```python
from build123d import *

# Parameters (mm, degrees)
SKETCH_2_W          = 308
SKETCH_2_H          = 840
EXTRUDE_1_DEPTH     = 1
SKETCH_2_3_W        = 22
SKETCH_2_3_H        = 840
EXTRUDE_2_DEPTH     = 22
SKETCH_4_W          = 20
SKETCH_4_H          = 20
CUT_EXTRUDE_1_DEPTH = 840
SKETCH_4_3_W        = 20
SKETCH_4_3_H        = 20
CUT_EXTRUDE_2_DEPTH = 840


with BuildPart() as part:
    # 스케치2 → 보스-돌출1 (new body)
    with BuildSketch(Plane.XY):
        with Locations((-176, 420)):
            Rectangle(SKETCH_2_W, SKETCH_2_H)
    extrude(amount=EXTRUDE_1_DEPTH)

    # 스케치2<3> → 보스-돌출2 (add)
    with BuildSketch(Plane.XY):
        with Locations((-11, 420)):
            Rectangle(SKETCH_2_3_W, SKETCH_2_3_H)
        with Locations((-341, 420)):
            Rectangle(SKETCH_2_3_W, SKETCH_2_3_H)
    extrude(amount=EXTRUDE_2_DEPTH)

    # 스케치4 → 컷-돌출1 (cut)
    with BuildSketch(Plane(origin=(0, 840, 0), x_dir=(1, 0, 0), z_dir=(0, 1, 0))):
        with Locations((-11, -11)):
            Rectangle(SKETCH_4_W, SKETCH_4_H)
    extrude(amount=-CUT_EXTRUDE_1_DEPTH, mode=Mode.SUBTRACT)

    # 스케치4<3> → 컷-돌출2 (cut)
    with BuildSketch(Plane(origin=(0, 840, 0), x_dir=(1, 0, 0), z_dir=(0, 1, 0))):
        with Locations((-341, -11)):
            Rectangle(SKETCH_4_3_W, SKETCH_4_3_H)
    extrude(amount=-CUT_EXTRUDE_2_DEPTH, mode=Mode.SUBTRACT)


solid = part.part
```
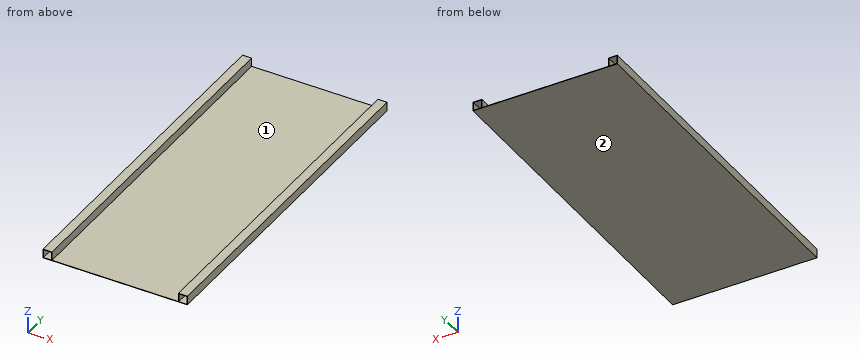
Check sheet for the modelled part. Datum: model origin and axes. Units: mm. Face numbers are marked on the shaded views. Give positions to 0.01 mm unless a question says otherwise; leave off trailing zeros. Order: outer loops, then holes, each group sorted by start corner. A loop starts at its lowest first (then second) coordinate and runs counter-clockwise, first axis right, second up. Notation, with made-up numbers: M 73.5,50 L 131.5,50 A24 cw 131.5,70 Z; hole C 30.5,26.5 d7. An arc over 180 degrees is marked long. Answer in a Markdown table with one row per item. Add a question column.
Q1. Thickness scan on L1, parallel to X at y = 161.5, z = 6; L2, parallel to Z at x = -142, y = 180.5. Record the ranges inside material, lowest first.
Q2. Release check for a two-part mould opening along X. For the marked faces 1 and 2 record: released by +X, released by -X, zero draft, split by the parting line, or undercut.
Q3. Sectioned sample at C-C, the plane x = -83.5. Record the boundary of the cut face in (y, z).
Q4. Sectioned sample at B-B, the plane y = 280. Record the boundary of the cut face in (x, z).
Q5. Gauge pin test, flat ends, axial feed: pin 1 Ø6 at (y, z) = (501.5, 7.5) entering from +X; pin 2 Ø10 at (x, y) = (-101.5, 124) entering from +Z. Record the tip position at first contact, or that the pin passes through.
Q6. Sectioned sample at A-A, the plane z = 8.5. Record the boundary of the cut face in (x, y), and give its area (3 significant figures).
Verdict:
| question | item | result |
|---|---|---|
| 1 | L1 | -352 to -351, -331 to -330, -22 to -21, -1 to 0 |
| 1 | L2 | 0 to 1 |
| 2 | face 1 | undercut |
| 2 | face 2 | zero draft |
| 3 | outline | M 0,0 L 840,0 L 840,1 L 0,1 Z |
| 4 | outline | M -352,0 L 0,0 L 0,22 L -22,22 L -22,1 L -330,1 L -330,22 L -352,22 Z; hole M -351,1 L -331,1 L -331,21 L -351,21 Z; hole M -21,1 L -1,1 L -1,21 L -21,21 Z |
| 5 | pin 1 | x = 0 |
| 5 | pin 2 | z = 1 |
| 6 | outline | M -352,0 L -351,0 L -351,840 L -352,840 Z; M -331,0 L -330,0 L -330,840 L -331,840 Z; M -22,0 L -21,0 L -21,840 L -22,840 Z; M -1,0 L 0,0 L 0,840 L -1,840 Z |
| 6 | area | 3,360 mm² |
